Autodesk Inventor part; units mm, degrees
ref_plane "YZ Plane" through (0, 0, 0) normal (1, 0, 0) x (0, 1, 0)
ref_plane "XZ Plane" through (0, 0, 0) normal (0, 1, 0) x (-1, 0, 0)
ref_plane "XY Plane" through (0, 0, 0) normal (0, 0, 1) x (1, 0, 0)
sketch "Sketch1" plane through (0, 0, 0) normal (0, 0, 1) x (1, 0, 0)
  circle A0 centre (0, 0) radius 30.734
  line L0 (-120.65, -78.74) -> (120.65, -78.74)
  line L1 (120.65, -78.74) -> (120.65, 48.26)
  line L2 (90.17, 78.74) -> (-90.17, 78.74)
  line L3 (-120.65, 48.26) -> (-120.65, -78.74)
  arc A1 (-90.17, 78.74) -> (-120.65, 48.26) centre (-90.17, 48.26) ccw
  arc A2 (120.65, 48.26) -> (90.17, 78.74) centre (90.17, 48.26) ccw
  point P0 (120.65, 78.74)
  point P1 (-120.65, 78.74)
  dimension "d0" = 61.468
  dimension "d1" = 157.48
  dimension "d2" = 241.3
  dimension "d3" = 78.74
  dimension "d4" = 120.65
  dimension "d5" = 30.48
extrude "Extrusion1" add sketch "Sketch1" against normal blind 187.96
sketch "Sketch2" plane through (0, 0, -187.96) normal (0, 0, -1) x (-1, 0, 0)
  circle A0 centre (0, 0) radius 30.734
  circle A1 centre (0, 0) radius 52.0012
extrude "Extrusion2" add sketch "Sketch2" against normal blind 127 contours A0 | A1
sketch "Sketch3" plane through (-120.65, -78.74, 0) normal (-1, 0, 0) x (0, 0, 1)
  line L0 (-187.96, 0) -> (-187.96, 127)
  line L1 (-187.96, 127) -> (-58.42, 127)
  line L2 (-58.42, -30.48) -> (-58.42, -215.9)
  line L3 (-58.42, -215.9) -> (-187.96, -215.9)
  line L4 (-187.96, -215.9) -> (-187.96, 127)
  line L5 (0, 0) -> (-187.96, 0)
  line L6 (-27.94, 0) -> (0, 0)
  line L7 (-187.96, -215.9) -> (-58.42, -215.9)
  line L8 (-58.42, -215.9) -> (-58.42, -30.48)
  line L9 (-58.42, 0) -> (-187.96, 0)
  line L10 (-187.96, 0) -> (-187.96, -215.9)
  arc A0 (-27.94, 0) -> (-58.42, -30.48) centre (-27.94, -30.48) ccw
  line L11 (0, 0) -> (-187.96, 0)
  line L12 (-187.96, -215.9) -> (-58.42, -215.9)
  arc A1 (-27.94, 0) -> (-58.42, -30.48) centre (-27.94, -30.48) ccw
  line L13 (-58.42, -30.48) -> (-58.42, -215.9)
  line L14 (-187.96, -215.9) -> (-187.96, 0)
  line L15 (-187.96, 0) -> (-27.94, 0)
  arc A2 (-27.94, 0) -> (-58.42, -30.48) centre (-27.94, -30.48) ccw
  point P0 (0, 78.74)
  dimension "d10" = 129.54
  dimension "d11" = 342.9
  dimension "d12" = 30.48
extrude "Extrusion3" add sketch "Sketch3" against normal blind 114.3
fillet "Fillet1" radius 30.48 1 edges at (-6.35, -78.74, -107.95)
sketch "Sketch4" plane through (-120.65, -78.74, 0) normal (-1, 0, 0) x (0, 0, 1)
  line L0 (0, 127) -> (-187.96, 127)
  line L1 (-187.96, 127) -> (-187.96, 69.85)
  line L2 (-187.96, 127) -> (-187.96, 0)
  line L3 (-144.78, 78.74) -> (-114.3, 78.74)
  circle A0 centre (-114.3, 78.74) radius 30.48
  line L4 (0, 127) -> (0, 0)
  point P0 (0, 78.74)
  dimension "d18" = 60.96
  dimension "d21" = 114.3
  dimension "d25" = 0
extrude "Extrusion4" add sketch "Sketch4" along normal blind 35.56
sketch "Sketch5" plane through (120.65, -78.74, 0) normal (1, 0, 0) x (0, 0, -1)
  line L0 (-23.8125, -17.4625) -> (228.6, -17.4625)
  line L1 (228.6, -17.4625) -> (228.6, 187.325)
  line L2 (228.6, 187.325) -> (-23.8125, 187.325)
  line L3 (-23.8125, 187.325) -> (-23.8125, -17.4625)
  point P0 (0, 78.74)
extrude "Extrusion5" cut sketch "Sketch5" against normal blind 63.5
fillet "Fillet2" radius 30.48 1 edges at (57.15, 78.74, -93.98)
equation "\"d3\" = 0.5 * d1"
properties part number "Shoulder1 Link"
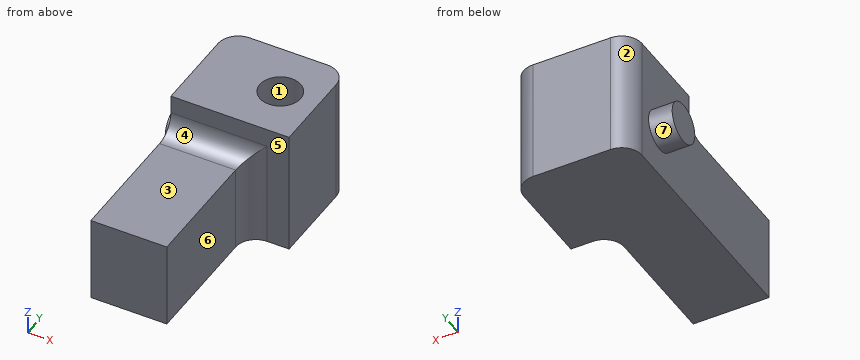
The listing builds one solid part. Answer for the finished solid, in the listing's coordinates (mm). Face numbers are marked on the shaded views. A direction names the side the tool comes from. Give positions to 0.01 mm unless a question says otherwise; leave off trailing zeros. Order: outer loops, then holes, each group sorted by start corner. A loop starts at its lowest first (then second) coordinate and runs counter-clockwise, first axis right, second up. Notation, with made-up numbers: (48, -20) -> (76, -20) arc R25 ccw to (76, 13) -> close; hole circle Ø7 at (41, 6). An arc over 180 degrees is marked (long way). One line per item, written item: value.
1) Find section B-B, the plane z = -114.3. Determine the outline of the cut face in (x, y), plus the area to 3 significant figures.
Reported:
outline: (-156.21, -30.48) -> (-120.65, -30.48) -> (-120.65, -294.64) -> (-6.35, -294.64) -> (-6.35, -109.22) arc R30.48 cw to (24.13, -78.74) -> (57.15, -78.74) -> (57.15, 48.26) arc R30.48 ccw to (26.67, 78.74) -> (-90.17, 78.74) arc R30.48 ccw to (-120.65, 48.26) -> (-120.65, 30.48) -> (-156.21, 30.48) -> close
area: 54,600 mm^2
2) Flat-ended cylindrical pins translate along their axes: P1, Ø1, axis at x = 4.5, z = -34, coming from the -Y side; P2, Ø3, axis at y = -82, z = -157, coming from the -X side; P3, Ø5, axis at x = -96.5, z = -79.5, coming from the +Y side. Find the tip coordinate at first contact, or state that the pin passes through.
Reported:
P1: stops at y = -79.45
P2: stops at x = -120.65
P3: stops at y = 78.5
3) Find section A-A, the plane x = -75.5. Determine the outline of the cut face in (y, z).
Reported:
outline: (-294.64, -187.96) -> (78.74, -187.96) -> (78.74, 0) -> (-78.74, 0) -> (-78.74, -27.94) arc R30.48 cw to (-109.22, -58.42) -> (-294.64, -58.42) -> close
4) Find the intervals of material crossed by line 1 (X direction, y = -274.5, z = -137.5); line 2 (X direction, y = 39, z = -32); line 3 (Y direction, x = 0, z = -20.5), in increasing order.
Reported:
line 1: x = -120.65 to -6.35
line 2: x = -120.65 to 57.15
line 3: y = -78.74 to -30.73, 30.73 to 78.74
5) Find section D-D, the plane z = -160. Determine the outline of the cut face in (x, y).
Reported:
outline: (-120.65, -294.64) -> (-6.35, -294.64) -> (-6.35, -109.22) arc R30.48 cw to (24.13, -78.74) -> (57.15, -78.74) -> (57.15, 48.26) arc R30.48 ccw to (26.67, 78.74) -> (-90.17, 78.74) arc R30.48 ccw to (-120.65, 48.26) -> close
6) Find section C-C, the plane y = -25. Determine the outline of the cut face in (x, z), plus the area to 3 significant figures.
Reported:
outline: (-156.21, -131.74) -> (-120.65, -131.74) -> (-120.65, -187.96) -> (57.15, -187.96) -> (57.15, 0) -> (17.88, 0) -> (17.88, -60.96) -> (-17.88, -60.96) -> (-17.88, 0) -> (-120.65, 0) -> (-120.65, -96.86) -> (-156.21, -96.86) -> close
area: 32,500 mm^2
7) A tool of negligible diameter and unlimited length cuts with its end or side. For the marked faces 5, 6 and 7, from which of +Z, -Z, +X, -X, +Y, -Y can it reach the whole face along a straight path? Write none if from no direction.
Reported:
face 5: +Z, +X, -Y
face 6: +Z, -Z, +X, -Y
face 7: -X
8) Determine the mould class of the marked faces 1, 2, 3 and 4 for opening direction Y: pulls with the +Y half, pulls with the -Y half, needs draft (parallel to the pull), parting line crosses it, or undercut.
Reported:
face 1: undercut
face 2: pulls with the +Y half
face 3: needs draft
face 4: pulls with the -Y half
